```python
from build123d import *

# Parameters (mm, degrees)
F0_R         = 25.3224131448
F0_R_2       = 25.3609127301
F1_DEPTH     = 11.176
F2_T1_DEPTH  = 4.1998379789
F2_T3_DEPTH  = 127.4783204379
F2_T5_DEPTH  = 4.1998416744
F2_T7_DEPTH  = 127.4783167424
F2_T10_ANGLE = 90
F2_T12_ANGLE = 90
F2_T14_ANGLE = 90
F2_T16_ANGLE = 90


# Not quite as in the source:
# - a fillet or chamfer that OpenCascade refuses, or shapes differently, is made with other operations: its cross-section is extruded or revolved along the edge and cut away or added


with BuildPart() as f1:
    # F0 (on Top) → F1 (new body)
    with BuildSketch(Plane.XY):
        with BuildLine():
            Line((70.0572131213, 37.4184697866), (-57.4211036211, 37.4184697866))
            ThreePointArc((-57.4211036211, 37.4184697866), (-74.0383517658, 30.5353802358), (-80.9214413166, 13.9181320912))
            Line((-80.9214413166, 13.9181320912), (-80.9214413166, 9.7182941123))
            ThreePointArc((-80.9214413166, 9.7182941123), (-74.0383528482, -6.8989514193), (-57.4211073166, -13.7820398877))
            Line((-57.4211073166, -13.7820398877), (70.0572131213, -13.7820398877))
            ThreePointArc((70.0572131213, -13.7820398877), (86.6744586529, -6.8989514193), (93.5575471213, 9.7182941123))
            Line((93.5575471213, 9.7182941123), (93.5575471213, 13.9181357866))
            ThreePointArc((93.5575471213, 13.9181357866), (86.6744586529, 30.5353813182), (70.0572131213, 37.4184697866))
        make_face()
        with Locations((-42.9976209998, 11.9247278199)):
            Circle(F0_R, mode=Mode.SUBTRACT)
        with Locations((57.7639937401, 11.9247278199)):
            Circle(F0_R_2, mode=Mode.SUBTRACT)
    extrude(amount=F1_DEPTH)

    # F2: fillet of radius 17.1698868556 on 1 edges, made by hand

    # F2_s2 → F2_t1 (cut)
    with BuildSketch(Plane.XZ.offset(-13.9181320912)):
        with BuildLine():
            ThreePointArc((-80.9214413166, 11.176), (-74.6269133611, 3.0681250194), (-64.8317447689, 0))
            Line((-64.8317447689, 0), (-64.8317447689, -0.3433977371))
            Line((-64.8317447689, -0.3433977371), (-80.9214413166, -0.3433977371))
            Line((-80.9214413166, -0.3433977371), (-81.2648390537, 0))
            ThreePointArc((-81.2648390537, 0), (-81.2648390537, 5.588), (-81.2432352476, 11.0561222629))
            Line((-81.2432352476, 11.0561222629), (-80.9214413166, 11.176))
        make_face()
    extrude(amount=F2_T1_DEPTH, mode=Mode.SUBTRACT)

    # F2_s4 → F2_t3 (cut)
    with BuildSketch(Plane.YZ.offset(-57.4211073166)):
        with BuildLine():
            ThreePointArc((-13.7820398877, 11.176), (-7.4875119322, 3.0681250194), (2.3076566599, 0))
            Line((2.3076566599, 0), (2.3076566599, -0.3433977371))
            Line((2.3076566599, -0.3433977371), (-13.7820398877, -0.3433977371))
            Line((-13.7820398877, -0.3433977371), (-14.1254376248, 0))
            ThreePointArc((-14.1254376248, 0), (-14.1254376248, 5.588), (-14.1038338187, 11.0561222629))
            Line((-14.1038338187, 11.0561222629), (-13.7820398877, 11.176))
        make_face()
    extrude(amount=F2_T3_DEPTH, mode=Mode.SUBTRACT)

    # F2_s6 → F2_t5 (cut)
    with BuildSketch(Plane.XZ.offset(-13.9181357866)):
        with BuildLine():
            ThreePointArc((93.5575471213, 11.176), (87.2630191658, 3.0681250194), (77.4678505736, 0))
            Line((77.4678505736, 0), (77.4678505736, -0.3433977371))
            Line((77.4678505736, -0.3433977371), (93.5575471213, -0.3433977371))
            Line((93.5575471213, -0.3433977371), (93.9009448584, 0))
            ThreePointArc((93.9009448584, 0), (93.9009448584, 5.588), (93.8793410523, 11.0561222629))
            Line((93.8793410523, 11.0561222629), (93.5575471213, 11.176))
        make_face()
    extrude(amount=F2_T5_DEPTH, mode=Mode.SUBTRACT)

    # F2_s8 → F2_t7 (cut)
    with BuildSketch(Plane.YZ.offset(-57.4211036211)):
        with BuildLine():
            ThreePointArc((37.4184697866, 11.176), (31.1239418311, 3.0681250194), (21.328773239, 0))
            Line((21.328773239, 0), (21.328773239, -0.3433977371))
            Line((21.328773239, -0.3433977371), (37.4184697866, -0.3433977371))
            Line((37.4184697866, -0.3433977371), (37.7618675238, 0))
            ThreePointArc((37.7618675238, 0), (37.7618675238, 5.588), (37.7402637176, 11.0561222629))
            Line((37.7402637176, 11.0561222629), (37.4184697866, 11.176))
        make_face()
    extrude(amount=F2_T7_DEPTH, mode=Mode.SUBTRACT)

    # F2_s9 → F2_t10 (revolve, cut)
    with BuildSketch(Plane.XZ.offset(-9.7182941123)):
        with BuildLine():
            ThreePointArc((-80.9214413166, 11.176), (-74.6269133611, 3.0681250194), (-64.8317447689, 0))
            Line((-64.8317447689, 0), (-64.8317447689, -0.3433977371))
            Line((-64.8317447689, -0.3433977371), (-80.9214413166, -0.3433977371))
            Line((-80.9214413166, -0.3433977371), (-81.2648390537, 0))
            ThreePointArc((-81.2648390537, 0), (-81.2648390537, 5.588), (-81.2432352476, 11.0561222629))
            Line((-81.2432352476, 11.0561222629), (-80.9214413166, 11.176))
        make_face()
    revolve(axis=Axis((-57.4211073166, 9.7182941123, 0), (0, 0, 1)), revolution_arc=F2_T10_ANGLE, mode=Mode.SUBTRACT)

    # F2_s11 → F2_t12 (revolve, cut)
    with BuildSketch(Plane.YZ.offset(70.0572131213)):
        with BuildLine():
            ThreePointArc((-13.7820398877, 11.176), (-7.4875119322, 3.0681250194), (2.3076566599, 0))
            Line((2.3076566599, 0), (2.3076566599, -0.3433977371))
            Line((2.3076566599, -0.3433977371), (-13.7820398877, -0.3433977371))
            Line((-13.7820398877, -0.3433977371), (-14.1254376248, 0))
            ThreePointArc((-14.1254376248, 0), (-14.1254376248, 5.588), (-14.1038338187, 11.0561222629))
            Line((-14.1038338187, 11.0561222629), (-13.7820398877, 11.176))
        make_face()
    revolve(axis=Axis((70.0572131213, 9.7182941123, 0), (0, 0, 1)), revolution_arc=F2_T12_ANGLE, mode=Mode.SUBTRACT)

    # F2_s13 → F2_t14 (revolve, cut)
    with BuildSketch(Plane.XZ.offset(-13.9181357866)):
        with BuildLine():
            ThreePointArc((93.5575471213, 11.176), (87.2630191658, 3.0681250194), (77.4678505736, 0))
            Line((77.4678505736, 0), (77.4678505736, -0.3433977371))
            Line((77.4678505736, -0.3433977371), (93.5575471213, -0.3433977371))
            Line((93.5575471213, -0.3433977371), (93.9009448584, 0))
            ThreePointArc((93.9009448584, 0), (93.9009448584, 5.588), (93.8793410523, 11.0561222629))
            Line((93.8793410523, 11.0561222629), (93.5575471213, 11.176))
        make_face()
    revolve(axis=Axis((70.0572131213, 13.9181357866, 0), (0, 0, 1)), revolution_arc=F2_T14_ANGLE, mode=Mode.SUBTRACT)

    # F2_s15 → F2_t16 (revolve, cut)
    with BuildSketch(Plane.YZ.offset(-57.4211036211)):
        with BuildLine():
            ThreePointArc((37.4184697866, 11.176), (31.1239418311, 3.0681250194), (21.328773239, 0))
            Line((21.328773239, 0), (21.328773239, -0.3433977371))
            Line((21.328773239, -0.3433977371), (37.4184697866, -0.3433977371))
            Line((37.4184697866, -0.3433977371), (37.7618675238, 0))
            ThreePointArc((37.7618675238, 0), (37.7618675238, 5.588), (37.7402637176, 11.0561222629))
            Line((37.7402637176, 11.0561222629), (37.4184697866, 11.176))
        make_face()
    revolve(axis=Axis((-57.4211036211, 13.9181320912, 0), (0, 0, 1)), revolution_arc=F2_T16_ANGLE, mode=Mode.SUBTRACT)


solid = f1.part
```
Read the model definition and answer for the solid it produces. Units are mm, in the model's axes. Coordinates: 2 decimals unless noted, no trailing zeros. Loops run counter-clockwise (first coordinate to the right, second up) from the corner with the lowest first, then second, coordinate; pieces in that order, holes last. Notation, with made-up numbers: (-5.5, 32.5) - (25.5, 32.5) arc R12 cw to (25.5, 44.5) - close; hole circle Ø11 at (-29.5, 7.25). An arc over 180 degrees is marked (long way). Answer in a Markdown table with one row per item.
1. Find section B-B, the plane y = -6. Count the separate pieces of the cut face and the enclosed holes in it, then the cut area to 3 significant figures.
Conclusion:
| item | result |
|---|---|
| separate pieces | 3 |
| enclosed holes | 0 |
| area | 738 mm² |
2. Find section D-D, the plane x = -55. Write down the section's boundary in (y, z).
Conclusion:
| item | result |
|---|---|
| outline | (-13.78, 11.18) arc R17.17 ccw to (-10.37, 5.59) - (-10.37, 11.18) - close; (34.22, 5.83) arc R17.17 ccw to (37.42, 11.18) - (34.22, 11.18) - close |
3. Find section A-A, the plane x = 66. Write down the section's boundary in (y, z).
Conclusion:
| item | result |
|---|---|
| outline | (-13.78, 11.18) arc R17.17 ccw to (-12.06, 7.77) - (-12.06, 11.18) - close; (35.91, 8.11) arc R17.17 ccw to (37.42, 11.18) - (35.91, 11.18) - close |
4. Given pin 1 (1.5 mm diameter, centred on x = 28, z = 4, fed in from -Y); pin 2 (6 mm diameter, centred on y = 24.5, z = 9.5, fed in from -X); pin 3 (4 mm diameter, centred on y = 31.5, z = 3.5, fed in from -X), each flat-ended and moving along its own axis, determine where each tip first touches the part or whether it passes through.
Conclusion:
| item | result |
|---|---|
| pin 1 | stops at y = -9.55 |
| pin 2 | stops at x = -79.48 |
| pin 3 | stops at x = -68.23 |
5. Determine the mould class of faces 1 (the face through (5, 12, 11.176)), 2 (the face through (-76.07, 11.85, 4.19)), 3 (the face through (37.64, -3.51, 6.75)) for opening direction X: +X half, -X half, draft (parallel to the pull), parting line (faces both ways), or undercut.
Conclusion:
| item | result |
|---|---|
| face 1 | draft |
| face 2 | -X half |
| face 3 | undercut |
6. Straight lines are drawn through the part: line 1 (X direction, y = 11, z = 6.75); line 2 (X direction, y = 20.5, z = 3.5); line 3 (Y direction, x = -26, z = 9.5). For each, find the intervals that lie inside material, in ascending order.
Conclusion:
| item | result |
|---|---|
| line 1 | x = -78.48 to -68.3, -17.69 to 32.42, 83.11 to 91.11 |
| line 2 | x = -73.96 to -66.82, -19.17 to 33.9, 81.63 to 86.6 |
| line 3 | y = -13.05 to -6.85, 30.69 to 36.69 |
